CAD build for the part. Positions are in the model's coordinates, mm. A direction names the side the tool comes from. Round coordinates to 2 decimals unless told otherwise and drop trailing zeros. Loops run counter-clockwise (first coordinate to the right, second up) from the corner with the lowest first, then second, coordinate; pieces in that order, holes last. Notation, with made-up numbers: M 38.5,-9.5 L 69.5,-9.5 A28 ccw 69.5,26.5 Z; hole C 69,24.5 d11. An arc over 180 degrees is marked long. Use one line per item in the form item = value.
from build123d import *

# Parameters (mm, degrees)
F0_R     = 37.5
F0_R_2   = 32.5
F1_DEPTH = 16
F2_W     = 14
F2_H     = 13.5
F3_DEPTH = 37.501
F4_W     = 15
F4_H     = 14.5
F5_DEPTH = 50
F6_R     = 60
F6_R_2   = 37.5
F6_R_3   = 32.5
F7_DEPTH = 3
F8_D     = 1.9
F8_DEPTH = 50
F8_TIP   = 0.5708175881
F9_D     = 4.4
F9_DEPTH = 50
F9_TIP   = 1.3218933619


with BuildPart() as f1:
    # F0 (on Top) → F1 (new body)
    with BuildSketch(Plane.XY):
        Circle(F0_R)
        Circle(F0_R_2, mode=Mode.SUBTRACT)
    extrude(amount=F1_DEPTH)

    # F2 (on Right) → F3 (cut, through all)
    with BuildSketch(Plane.YZ):
        with Locations((0, 6.75)):
            Rectangle(F2_W, F2_H)
    extrude(amount=-F3_DEPTH, mode=Mode.SUBTRACT)

    # F4 (on Front) → F5 (cut)
    with BuildSketch(Plane.XZ):
        with Locations((0, 7.25)):
            Rectangle(F4_W, F4_H)
    extrude(amount=F5_DEPTH, mode=Mode.SUBTRACT)

    # F6 (on face) → F7 (join)
    with BuildSketch(Plane.XY.offset(16)):
        Circle(F6_R)
        Circle(F6_R_2, mode=Mode.SUBTRACT)
        Circle(F6_R_2)
        Circle(F6_R_3, mode=Mode.SUBTRACT)
    extrude(amount=F7_DEPTH)

    # F8 (one way)
    with BuildSketch(Plane.XY.offset(16)):
        with Locations((32.3357836379, -13.3939201328), (13.3939201328, 32.3357836379), (-13.3939201328, -32.3357836379), (-32.3357836379, 13.3939201328), (-13.3939201328, 32.3357836379), (32.3357836379, 13.3939201328), (13.3939201328, -32.3357836379), (-32.3357836379, -13.3939201328)):
            Circle(F8_D / 2)
    extrude(amount=-F8_DEPTH, mode=Mode.SUBTRACT)
    with Locations(Plane.XY.offset(16)):
        with Locations((32.3357836379, -13.3939201328), (13.3939201328, 32.3357836379), (-13.3939201328, -32.3357836379), (-32.3357836379, 13.3939201328), (-13.3939201328, 32.3357836379), (32.3357836379, 13.3939201328), (13.3939201328, -32.3357836379), (-32.3357836379, -13.3939201328)):
            with Locations((0, 0, -(F8_DEPTH + F8_TIP / 2))):  # 118° drill point
                Cone(0, F8_D / 2, F8_TIP, mode=Mode.SUBTRACT)

    # F9
    with Locations(Plane(origin=(0, 0, 16), x_dir=(1, 0, 0), z_dir=(0, 0, -1))):
        with Locations((-36.0624458405, -36.0624458405), (36.0624458405, -36.0624458405), (36.0624458405, 36.0624458405), (-36.0624458405, 36.0624458405)):
            Hole(F9_D / 2, depth=F9_DEPTH)
            with Locations((0, 0, -(F9_DEPTH + F9_TIP / 2))):  # 118° drill point
                Cone(0, F9_D / 2, F9_TIP, mode=Mode.SUBTRACT)


solid = f1.part
1. Drop flat-ended pins along their axis: P1, Ø1.5, axis at x = -34, z = 7, coming from the -Y side; P2, Ø1, axis at y = -7.5, z = 10, coming from the +X side; P3, Ø1.5, axis at x = 27, z = 5.5, coming from the +Y side; P4, Ø4, axis at y = -40.5, z = 4, coming from the -X side. Give the stop position or say it passes through.
Completed:
P1 = -17.34
P2 = 36.84
P3 = 26.78
P4 = through
2. Cut at C-C on y = 0. Write the cut outline in (x, z).
Completed:
outline = M -60,16 L -37.5,16 L -37.5,13.5 L -32.5,13.5 L -32.5,19 L -60,19 Z; M 32.5,0 L 37.5,0 L 37.5,16 L 60,16 L 60,19 L 32.5,19 Z
3. Pull direction X, two halves, no side cores. Call faces 1 (the face through (37.808, -34.724, 17.521)), 2 (the face through (35.77, 11.26, 7.89)), 3 (the face through (-34, 7, 7)): +X half, -X half, draft (parallel to the pull), parting line (faces both ways), or undercut.
Completed:
face_1 = undercut
face_2 = parting line
face_3 = draft
4. Tool access for faces 4 (the face through (-34, -7, 7)), 5 (the face through (37.81, 37.4, 17.52)), 6 (the face through (-7.5, -34, 7)), 7 (the face through (26, 28, 16)): list every direction of +Z, -Z, +X, -X, +Y, -Y with a clear straight run to the whole face (end or side of a thin tool).
Completed:
face_4 = -Z, -X
face_5 = +Z, -Z
face_6 = -Z, -Y
face_7 = -Z
5. Probe line 1 along Y through (x, z) = (-33, 13); line 2 along Z through (x, y) = (-47, 36); line 3 along X through (y, z) = (25, 3). List the from-to ranges inside material, lowest first. Write a range as from..to.
Completed:
line_1 = -17.81..-14.07, -12.71..-7, 7..12.71, 14.07..17.81
line_2 = 16..19
line_3 = -27.95..-20.77, 20.77..27.95
6. Cut at A-A on x = 0. Write the cut outline in (y, z).
Completed:
outline = M -60,16 L -37.5,16 L -37.5,14.5 L -32.5,14.5 L -32.5,19 L -60,19 Z; M 32.5,0 L 37.5,0 L 37.5,16 L 60,16 L 60,19 L 32.5,19 Z
7. Cut at B-B on z = 7.75. State how many separate pieces and enclosed holes the cut face has, and give its area (3 significant figures).
Completed:
separate_pieces = 2
enclosed_holes = 8
area = 931 mm2
